```python
from build123d import *

# Parameters (mm, degrees)
SKETCH1_R           = 5.1
SKETCH1_R_2         = 4.6
BOSS_EXTRUDE1_DEPTH = 3
SKETCH2_R           = 7.6
SKETCH2_R_2         = 4.6
BOSS_EXTRUDE2_DEPTH = 7
FILLET1_R           = 10
FILLET2_R           = 3
SKETCH3_R           = 15
CUT_EXTRUDE1_DEPTH  = 7
CUT_EXTRUDE2_DEPTH  = 7


with BuildPart() as part:
    # Sketch1 → Boss-Extrude1 (new body)
    with BuildSketch(Plane(origin=(0, 0, 0), x_dir=(1, 0, 0), z_dir=(0, 1, 0))):
        with BuildLine():
            ThreePointArc((-42.589636172, 29.834927363), (-52, 0), (-42.589636172, -29.834927363))
            ThreePointArc((-42.589636172, -29.834927363), (-41.790010768, -41.790010768), (-29.834927363, -42.589636172))
            ThreePointArc((-29.834927363, -42.589636172), (0, -52), (29.834927363, -42.589636172))
            ThreePointArc((29.834927363, -42.589636172), (41.790010768, -41.790010768), (42.589636172, -29.834927363))
            ThreePointArc((42.589636172, -29.834927363), (52, 0), (42.589636172, 29.834927363))
            ThreePointArc((42.589636172, 29.834927363), (41.790010768, 41.790010768), (29.834927363, 42.589636172))
            ThreePointArc((29.834927363, 42.589636172), (0, 52), (-29.834927363, 42.589636172))
            ThreePointArc((-29.834927363, 42.589636172), (-41.790010768, 41.790010768), (-42.589636172, 29.834927363))
        make_face()
        with Locations(Location((-35.355339059, -35.355339059, 0), (0, 0, 270))):
            Circle(SKETCH1_R, mode=Mode.SUBTRACT)
        with Locations(Location((-29.455003079, -13.735093507, 0), (0, 0, 270))):
            Circle(SKETCH1_R_2, mode=Mode.SUBTRACT)
        with Locations(Location((15.636875684, -33.53338812, 0), (0, 0, 270))):
            Circle(SKETCH1_R_2, mode=Mode.SUBTRACT)
        with Locations(Location((35.355339059, -35.355339059, 0), (0, 0, 270))):
            Circle(SKETCH1_R, mode=Mode.SUBTRACT)
        with Locations(Location((33.53338812, -15.636875684, 0), (0, 0, 270))):
            Circle(SKETCH1_R_2, mode=Mode.SUBTRACT)
        with Locations(Location((-29.455003079, 13.735093507, 0), (0, 0, 270))):
            Circle(SKETCH1_R_2, mode=Mode.SUBTRACT)
        with Locations(Location((-35.355339059, 35.355339059, 0), (0, 0, 270))):
            Circle(SKETCH1_R, mode=Mode.SUBTRACT)
        with Locations(Location((35.355339059, 35.355339059, 0), (0, 0, 270))):
            Circle(SKETCH1_R, mode=Mode.SUBTRACT)
    extrude(amount=BOSS_EXTRUDE1_DEPTH)

    # Sketch2 → Boss-Extrude2 (add)
    # profile 1 of 4: a face of its own
    with BuildSketch(Plane(origin=(0, 3, 0), x_dir=(1, 0, 0), z_dir=(0, 1, 0))):
        with Locations(Location((-29.455003079, 13.735093507, 0), (0, 0, 270))):
            Circle(SKETCH2_R)
        with Locations(Location((-29.455003079, 13.735093507, 0), (0, 0, 270))):
            Circle(SKETCH2_R_2, mode=Mode.SUBTRACT)
    # profile 2 of 4: a face of its own
    with BuildSketch(Plane(origin=(0, 3, 0), x_dir=(1, 0, 0), z_dir=(0, 1, 0))):
        with Locations(Location((-29.455003079, -13.735093507, 0), (0, 0, 270))):
            Circle(SKETCH2_R)
        with Locations(Location((-29.455003079, -13.735093507, 0), (0, 0, 270))):
            Circle(SKETCH2_R_2, mode=Mode.SUBTRACT)
    # profile 3 of 4: a face of its own
    with BuildSketch(Plane(origin=(0, 3, 0), x_dir=(1, 0, 0), z_dir=(0, 1, 0))):
        with Locations(Location((15.636875684, -33.53338812, 0), (0, 0, 270))):
            Circle(SKETCH2_R)
        with Locations(Location((15.636875684, -33.53338812, 0), (0, 0, 270))):
            Circle(SKETCH2_R_2, mode=Mode.SUBTRACT)
    # profile 4 of 4: a face of its own
    with BuildSketch(Plane(origin=(0, 3, 0), x_dir=(1, 0, 0), z_dir=(0, 1, 0))):
        with Locations(Location((33.53338812, -15.636875684, 0), (0, 0, 270))):
            Circle(SKETCH2_R)
        with Locations(Location((33.53338812, -15.636875684, 0), (0, 0, 270))):
            Circle(SKETCH2_R_2, mode=Mode.SUBTRACT)
    extrude(amount=BOSS_EXTRUDE2_DEPTH)

    # Fillet1
    fillet1_edges = [part.edges().sort_by_distance(p)[0] for p in [
        (-42.589636172, 1.5, 29.834927363),
        (-42.589636172, 1.5, -29.834927363),
        (-29.834927363, 1.5, -42.589636172),
        (29.834927363, 1.5, -42.589636172),
        (42.589636172, 1.5, -29.834927363),
        (42.589636172, 1.5, 29.834927363),
        (29.834927363, 1.5, 42.589636172),
        (-29.834927363, 1.5, 42.589636172),
    ]]
    fillet(fillet1_edges, radius=FILLET1_R)

    # Fillet2
    fillet2_edges = [part.edges().sort_by_distance(p)[0] for p in [
        (-29.455003079, 3, -21.335093507),
        (-29.455003079, 3, 6.135093507),
        (15.636875684, 3, 25.93338812),
        (33.53338812, 3, 8.036875684),
    ]]
    fillet(fillet2_edges, radius=FILLET2_R)

    # Sketch3 → Cut-Extrude1 (cut)
    with BuildSketch(Plane(origin=(0, 3, 0), x_dir=(1, 0, 0), z_dir=(0, 1, 0))):
        with Locations(Location((0, 0, 0), (0, 0, 270))):
            Circle(SKETCH3_R)
    extrude(amount=-CUT_EXTRUDE1_DEPTH, mode=Mode.SUBTRACT)

    # Sketch4 → Cut-Extrude2 (cut)
    with BuildSketch(Plane(origin=(0, 3, 0), x_dir=(1, 0, 0), z_dir=(0, 1, 0))):
        with BuildLine():
            ThreePointArc((37.681674094, 13.715007747), (16.946992296, 36.34294226), (-13.715007747, 37.681674094))
            ThreePointArc((-13.715007747, 37.681674094), (-18.257318576, 27.940657086), (-8.516301569, 23.398346258))
            ThreePointArc((-8.516301569, 23.398346258), (10.523194717, 22.567063897), (23.398346258, 8.516301569))
            ThreePointArc((23.398346258, 8.516301569), (33.139363265, 3.97399074), (37.681674094, 13.715007747))
        make_face()
    extrude(amount=-CUT_EXTRUDE2_DEPTH, mode=Mode.SUBTRACT)


solid = part.part
```
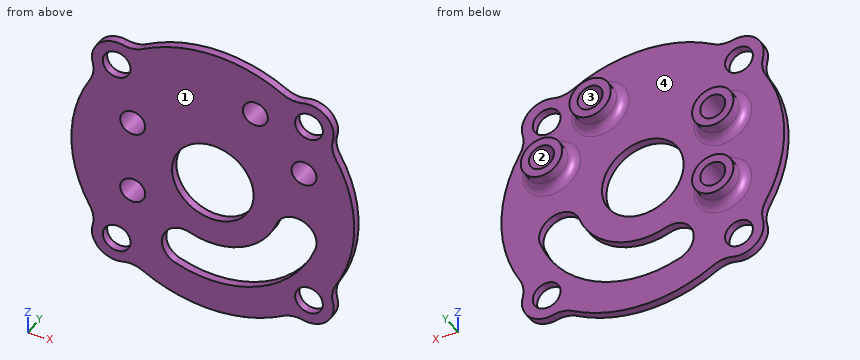
Can you work these out from the model? Positions are in its coordinate system, mm. Face numbers are marked on the shaded views. A direction names the side the tool comes from. Give positions to 0.01 mm unless a question says otherwise; leave off trailing zeros. Write each loop counter-clockwise with the first axis right and the second up, starting at its lowest first coordinate (ties: lowest second). Pieces come first, ordered by that corner, then holes. Notation, with made-up numbers: (53, 66) -> (57, 66) arc R12 cw to (57, 77) -> close; hole circle Ø2 at (-39, -31.75). An arc over 180 degrees is marked (long way). One line per item, written item: value.
Q1. Imagine slicing it at C-C on y = 7.5. Please give me the cut outline in (x, z) (3 decimals).
Results found:
outline: circle Ø15.2 at (-29.455, -13.735); circle Ø15.2 at (-29.455, 13.735); circle Ø15.2 at (15.637, 33.533); circle Ø15.2 at (33.533, 15.637); hole circle Ø9.2 at (-29.455, -13.735); hole circle Ø9.2 at (-29.455, 13.735); hole circle Ø9.2 at (15.637, 33.533); hole circle Ø9.2 at (33.533, 15.637)
Q2. Imagine slicing it at A-A on x = 0. Please give me the cut outline in (y, z).
Results found:
outline: (0, -52) -> (3, -52) -> (3, -40.1) -> (0, -40.1) -> close; (0, -24.9) -> (3, -24.9) -> (3, -15) -> (0, -15) -> close; (0, 15) -> (3, 15) -> (3, 52) -> (0, 52) -> close
Q3. We'd pull the mould along X, two halves only. Please class the marked faces 1 and 2: +X half, -X half, draft (parallel to the pull), parting line (faces both ways), or undercut.
Results found:
face 1: draft
face 2: undercut
Q4. Imagine slicing it at B-B on z = 0. Please give me the cut outline in (x, y), and give its area (3 significant figures).
Results found:
outline: (-52, 0) -> (-15, 0) -> (-15, 3) -> (-52, 3) -> close; (15, 0) -> (52, 0) -> (52, 3) -> (15, 3) -> close
area: 222 mm^2
Q5. For P1, Ø16.5, axis at x = 35.36, z = 35.36, coming from the +Y side; P2, Ø3, axis at x = 34.5, y = 6, coming from the +Z side, each with a flat end and sliding along its axis, tell me the tip position at first contact or that it passes through.
Results found:
P1: stops at y = 3
P2: stops at z = 23.59
Q6. Please list where these lines run through material, in increasing order: line 1 (X direction, y = 0.5, z = 37); line 2 (X direction, y = 2.5, z = -12.5); line 3 (Z direction, x = 39.5, y = 0.5). Write a range as [from, to].
Results found:
line 1: x = [-44.31, -40.18], [-30.53, 12.61], [18.66, 30.53], [40.18, 44.31]
line 2: x = [-50.48, -33.89], [-25.02, -8.29], [8.29, 21.54], [38.01, 50.48]
line 3: z = [-43.46, -38.33], [-32.38, 32.38], [38.33, 43.46]
Q7. Which directions (+Z, -Z, +X, -X, +Y, -Y) give clear straight access to the entire face, cutting with the end or side of a thin tool? Please do the marked faces 3 and 4.
Results found:
face 3: +Y, -Y
face 4: +Y
Q8. Imagine slicing it at D-D on z = 17. Give the number of separate pieces and of enclosed holes in the cut face, and give its area (3 significant figures).
Results found:
separate pieces: 3
enclosed holes: 0
area: 351 mm^2
